from build123d import *

# Parameters (mm, degrees)
SKETCH1_R           = 2.8
BOSS_EXTRUDE1_DEPTH = 5
CUT_EXTRUDE1_DEPTH  = 2.5
FILLET1_R           = 1.2


with BuildPart() as part:
    # Sketch1 → Boss-Extrude1 (new body)
    with BuildSketch(Plane.XY.offset(10)):
        with BuildLine():
            Line((-253, 240), (-241, 240))
            Line((-241, 240), (-241, 233.219543457))
            ThreePointArc((-241, 233.219543457), (-235.964643127, 224), (-241, 214.780456543))
            Line((-241, 214.780456543), (-241, 208))
            Line((-241, 208), (-253, 208))
            Line((-253, 208), (-253, 214.780456543))
            ThreePointArc((-253, 214.780456543), (-258.20228405, 224), (-253, 233.219543457))
            Line((-253, 233.219543457), (-253, 240))
        make_face()
        with Locations((-246.922635101, 224)):
            Circle(SKETCH1_R, mode=Mode.SUBTRACT)
    extrude(amount=BOSS_EXTRUDE1_DEPTH)

    # Sketch2 → Cut-Extrude1 (cut)
    with BuildSketch(Plane.XY.offset(15)):
        Polygon((-249.671711, 236.526764937), (-244.414971283, 236.526764937), (-244.414971283, 226.843297037), (-237.940881316, 226.843297037), (-237.940881316, 221.752559627), (-243.750962055, 221.752559627), (-243.750962055, 211.604094919), (-249.671711, 211.604094919), (-249.671711, 221.752559627), (-256.108895334, 221.752559627), (-256.108895334, 226.843297037), (-249.671711, 226.843297037), align=None)
    extrude(amount=-CUT_EXTRUDE1_DEPTH, mode=Mode.SUBTRACT)

    # Fillet1
    fillet1_edges = [part.edges().sort_by_distance(p)[0] for p in [
        (-249.671711, 226.843297037, 13.75),
        (-249.671711, 236.526764937, 13.75),
        (-244.414971283, 236.526764937, 13.75),
        (-244.414971283, 226.843297037, 13.75),
        (-237.940881316, 226.843297037, 13.75),
        (-237.940881316, 221.752559627, 13.75),
        (-243.750962055, 221.752559627, 13.75),
        (-243.750962055, 211.604094919, 13.75),
        (-249.671711, 211.604094919, 13.75),
        (-249.671711, 221.752559627, 13.75),
        (-256.108895334, 221.752559627, 13.75),
        (-256.108895334, 226.843297037, 13.75),
    ]]
    fillet(fillet1_edges, radius=FILLET1_R)


solid = part.part
Could you check a few things on this model? Use its own coordinates, in mm. A direction names the side the tool comes from. Give positions to 0.01 mm unless a question says otherwise; leave off trailing zeros. Order: outer loops, then holes, each group sorted by start corner. A loop starts at its lowest first (then second) coordinate and runs counter-clockwise, first axis right, second up.
1. Suppose I cut it at B-B (y = 224). List the corners of the cut face in (x, z) for me, plus the area to 3 significant figures.
2. For faces 1 (the flat face through (-253, 211, 12)), 2 (the flat face through (-247, 236.527, 14)), 3 (the cylindrical face through (-235.966, 224.153, 12.465)), which set-ups out of +Z, -Z, +X, -X, +Y, -Y let a thin tool reach every point of the face, with its end or its side?
3. Suppose I cut it at D-D (x = -252.5). List the corners of the cut face in (y, z) for me, plus the area to 3 significant figures.
4. Will these pins go through, and if not, where does the flat tip stop? P1, Ø2, axis at y = 217, z = 14, coming from the -X side; P2, Ø3, axis at y = 232, z = 14.5, coming from the -X side; P3, Ø1.5, axis at y = 213, z = 12.5, coming from the -X side.
5. I need wall thicknesses on L1, parallel to X at y = 224, z = 11.25; L2, parallel to X at y = 233.5, z = 14.05; L3, parallel to Y at x = -251.75, z = 14.7. Which ranges of each line are inside material? Lowest first, please.
6. Suppose I cut it at A-A (z = 11.4). List the corners of the cut face in (x, y) for me, plus the area to 3 significant figures.
7. Suppose I cut it at C-C (x = -246.5). List the corners of the cut face in (y, z) for me, plus the area to 3 significant figures.
8. We'd pull the mould along Y, two halves only. Please class faces 4 (the flat face through (-253, 226.843, 14)), 5 (the flat face through (-247, 240, 12)), 6 (the flat face through (-253, 237, 12)): pulls with the +Y half, pulls with the -Y half, needs draft (parallel to the pull), parting line crosses it, or undercut.
Solved:
1. outline: (-258.2, 10) - (-249.72, 10) - (-249.72, 12.5) - (-256.11, 12.5) - (-256.11, 15) - (-258.2, 15) - close; (-244.12, 10) - (-235.96, 10) - (-235.96, 15) - (-237.94, 15) - (-237.94, 12.5) - (-244.12, 12.5) - close
1. area: 51.8 mm2
2. face 1: +Z, -Z, -X, -Y
2. face 2: +Z
2. face 3: +Z, -Z, +X
3. outline: (208, 10) - (240, 10) - (240, 15) - (226.84, 15) - (226.84, 12.5) - (221.75, 12.5) - (221.75, 15) - (208, 15) - close
3. area: 147 mm2
4. P1: stops at x = -256.38
4. P2: stops at x = -256.02
4. P3: stops at x = -253
5. L1: x = -258.2 to -249.72, -244.12 to -235.96
5. L2: x = -253 to -249.67, -244.41 to -241
5. L3: y = 208 to 221.75, 226.84 to 240
6. outline: (-253, 208) - (-241, 208) - (-241, 214.78) arc R10.96 ccw to (-241, 233.22) - (-241, 240) - (-253, 240) - (-253, 233.22) arc R10.77 ccw to (-253, 214.78) - close; hole circle Ø5.6 at (-246.92, 224)
6. area: 493 mm2
7. outline: (208, 10) - (221.23, 10) - (221.23, 12.5) - (211.6, 12.5) - (211.6, 15) - (208, 15) - close; (226.77, 10) - (240, 10) - (240, 15) - (236.53, 15) - (236.53, 12.5) - (226.77, 12.5) - close
7. area: 83.9 mm2
8. face 4: undercut
8. face 5: pulls with the +Y half
8. face 6: needs draft
